Autodesk Inventor part; units mm, degrees
ref_plane "YZ Plane" through (0, 0, 0) normal (1, 0, 0) x (0, 1, 0)
ref_plane "XZ Plane" through (0, 0, 0) normal (0, 1, 0) x (-1, 0, 0)
ref_plane "XY Plane" through (0, 0, 0) normal (0, 0, 1) x (1, 0, 0)
sketch "Esquisse1" plane through (0, 0, 0) normal (1, 0, 0) x (0, 1, 0)
  line L0 (0, 0) -> (5, 0)
  line L1 (5, 0) -> (5, -30)
  line L2 (5, -30) -> (0, -30)
  line L3 (0, -30) -> (0, 0)
  dimension "d0" = 5
  dimension "d1" = 30
extrude "Extrusion1" add sketch "Esquisse1" along normal blind 10
sketch "Esquisse2" plane through (0, 5, 0) normal (0, 1, 0) x (1, 0, 0)
  line L0 (0, 0) -> (5, 0)
  line L1 (0, 0) -> (10, 0)
  line L2 (5, 0) -> (5, 8)
  arc A0 (1.4921, 8.545) -> (8.5079, 8.545) centre (5, 8) ccw
  line L3 (5, 21.75) -> (5, 20.05)
  arc A1 (6.6798, 20.311) -> (3.3202, 20.311) centre (5, 20.05) ccw
  line L4 (1.4921, 8.545) -> (3.3202, 20.311)
  line L5 (8.5079, 8.545) -> (6.6798, 20.311)
  line L6 (5, 4.45) -> (5, 11.55)
  line L7 (5, 18.35) -> (5, 21.75)
  dimension "d4" = 8
  dimension "d5" = 7.1
  dimension "d6" = 17.3
  dimension "d7" = 1.7
extrude "Extrusion2" cut sketch "Esquisse2" against normal blind 3.5
sketch "Esquisse3" plane through (0, 5, 0) normal (0, 1, 0) x (1, 0, 0)
  arc A0 (1.4921, 8.545) -> (8.5079, 8.545) centre (5, 8) ccw
  arc A1 (8.4161, 9.1358) -> (1.5839, 9.1358) centre (5, 8) ccw
  arc A2 (6.6798, 20.311) -> (3.3202, 20.311) centre (5, 20.05) ccw
  arc A3 (6.6798, 20.311) -> (3.3202, 20.311) centre (5, 20.05) ccw
  line L0 (1.4921, 8.545) -> (3.3202, 20.311)
  line L1 (3.3202, 20.311) -> (1.4921, 8.545)
  line L2 (6.6798, 20.311) -> (8.5079, 8.545)
  point P0 (0, 0)
  dimension "d24" = 7.2
extrude "Extrusion5" add sketch "Esquisse3" against normal blind 1.4 contours L0 A2 L2 A1
sketch "Esquisse5" plane through (0, 5, 0) normal (0, 1, 0) x (1, 0, 0)
  arc A0 (1.4921, 8.545) -> (8.5079, 8.545) centre (5, 8) ccw
  line L0 (5, 0) -> (1.45, 0)
  line L1 (0, 0) -> (10, 0)
  line L2 (1.45, 0) -> (1.45, 8)
  line L3 (1.45, 8) -> (8.55, 8)
  line L4 (8.55, 8) -> (8.55, 0)
  line L5 (8.55, 0) -> (1.45, 0)
  line L6 (5, 8) -> (5, 0)
  dimension "d27" = 3.55
  dimension "d28" = 7.1
extrude "Extrusion6" cut sketch "Esquisse5" against normal blind 3.5
sketch "Esquisse6" plane through (0, 5, 0) normal (0, 1, 0) x (1, 0, 0)
  arc A0 (8.4161, 9.1358) -> (1.5839, 9.1358) centre (5, 8) ccw
  line L0 (5, 8) -> (5, 0)
  line L1 (5, 0) -> (1.55, 0)
  line L2 (0, 0) -> (10, 0)
  line L3 (1.55, 0) -> (1.55, 6.5)
  line L4 (8.45, 6.5) -> (8.45, 0)
  line L5 (8.45, 0) -> (1.55, 0)
  line L6 (8.55, 8) -> (8.55, 0)
  line L7 (8.45, 6.5) -> (8.55, 6.5)
  line L8 (8.55, 6.5) -> (8.55, 0)
  line L9 (8.55, 0) -> (8.45, 0)
  line L10 (8.45, 0) -> (8.45, 6.5)
  line L11 (1.45, 0) -> (1.45, 8)
  line L12 (1.55, 6.5) -> (1.45, 6.5)
  line L13 (1.45, 6.5) -> (1.45, 0)
  line L14 (1.45, 0) -> (1.55, 0)
  line L15 (1.55, 0) -> (1.55, 6.5)
  dimension "d31" = 3.45
  dimension "d32" = 6.5
  dimension "d33" = 6.9
  dimension "d34" = 6.5
extrude "Extrusion8" add sketch "Esquisse6" against normal blind 1.5
sketch "Esquisse7" plane through (0, 0, -30) normal (0, -1, 0) x (1, 0, 0)
  line L0 (0, 0) -> (10, 0)
  line L1 (10, 0) -> (10, -105)
  line L2 (10, -105) -> (0, -105)
  line L3 (0, -105) -> (0, 0)
  point P0 (0, 30)
  dimension "d39" = 10
  dimension "d40" = 105
extrude "Extrusion9" add sketch "Esquisse7" against normal blind 5
properties part number "Barrière"
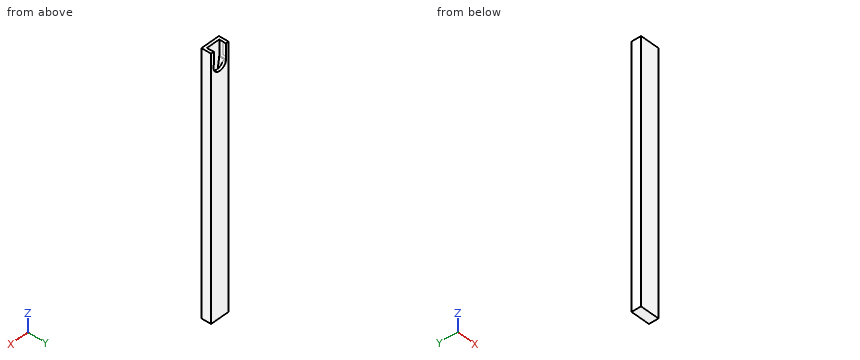
CAD build for the part. Positions are in the model's coordinates, mm. Round coordinates to 2 decimals unless told otherwise and drop trailing zeros. Loops run counter-clockwise (first coordinate to the right, second up) from the corner with the lowest first, then second, coordinate; pieces in that order, holes last. Notation, with made-up numbers: M 18.25,-33.5 L 48.25,-33.5 A19 cw 48.25,3.5 Z; hole C -23.75,-39.5 d3. An arc over 180 degrees is marked long. Use a Markdown table: item, result. Add a question column.
(1) Cut at B-B (y = 2.5). Give the cut face in (x, z) (3 decimals), and give its area (3 significant figures).
(2) Flat gauge pin, fed straight in: pin 1 (1 mm diameter, centred on y = 4, z = -76.5, fed in from -X). Where does the tip first touch, or does it go through?
(3) Cut at A-A (x = 4.5). Give the cut face in (y, z).
(4) Drill centre lines: line 1 (Y direction, x = 6.5, z = -17); line 2 (Z direction, x = 6, y = 4.75); line 3 (Z direction, x = 4, y = 2.4). Where is each one in solid material? Low to high.
Geometry says:
| question | item | result |
|---|---|---|
| 1 | outline | M 0,-135 L 10,-135 L 10,0 L 8.55,0 L 8.55,-8 A3.55 cw 8.508,-8.545 L 6.68,-20.311 A1.7 cw 3.32,-20.311 L 1.492,-8.545 A3.55 cw 1.45,-8 L 1.45,0 L 0,0 Z |
| 1 | area | 1,220 mm² |
| 2 | pin 1 | stops at x = 0 |
| 3 | outline | M 0,-135 L 5,-135 L 5,-11.57 L 3.6,-11.57 L 3.6,-21.67 L 1.5,-21.67 L 1.5,0 L 0,0 Z |
| 4 | line 1 | y = 0 to 1.5, 3.6 to 5 |
| 4 | line 2 | z = -135 to -11.46 |
| 4 | line 3 | z = -135 to -21.42 |
